```python
from build123d import *

# Parameters (mm, degrees)
F1_DEPTH = 40.2336
F2_DEPTH = 15.7734
F3_R     = 3.302


with BuildPart() as f1:
    # F0 (on Top) → F1 (new body)
    with BuildSketch(Plane.XY):
        with BuildLine():
            ThreePointArc((15.4849246273, -24.0155727453), (25.0899616005, -13.6756883515), (28.575, 0))
            ThreePointArc((28.575, 0), (24.3073468487, 15.0227665288), (12.7791284914, 25.5582569828))
            ThreePointArc((12.7791284914, 25.5582569828), (-28.532530963, -1.5573380643), (15.4849246273, -24.0155727453))
        make_face()
        with BuildLine():
            Line((18.5293, 4.826), (18.5293, 0))
            Line((18.5293, 0), (18.5293, -4.826))
            Line((18.5293, -4.826), (13.4477648793, -4.826))
            ThreePointArc((13.4477648793, -4.826), (-14.2875, 0), (13.4477648793, 4.826))
            Line((13.4477648793, 4.826), (18.5293, 4.826))
        make_face(mode=Mode.SUBTRACT)
    extrude(amount=F1_DEPTH)

    # F0 (on Top) → F2 (join)
    with BuildSketch(Plane.XY):
        with BuildLine():
            ThreePointArc((12.7791284914, 25.5582569828), (24.3073468487, 15.0227665288), (28.575, 0))
            Line((28.575, 0), (40.005, 0))
            ThreePointArc((40.005, 0), (44.0967182668, 9.8782817332), (53.975, 13.97))
            Line((53.975, 13.97), (12.7791284914, 25.5582569828))
        make_face()
        with BuildLine():
            Line((40.005, 0), (28.575, 0))
            ThreePointArc((28.575, 0), (25.0899616005, -13.6756883515), (15.4849246273, -24.0155727453))
            Line((15.4849246273, -24.0155727453), (53.975, -13.97))
            ThreePointArc((53.975, -13.97), (44.0967182668, -9.8782817332), (40.005, 0))
        make_face()
        with BuildLine():
            Line((46.355, 0), (40.005, 0))
            ThreePointArc((40.005, 0), (44.0967182668, -9.8782817332), (53.975, -13.97))
            Line((53.975, -13.97), (53.975, -7.62))
            ThreePointArc((53.975, -7.62), (48.5868463274, -5.3881536726), (46.355, 0))
        make_face()
        with BuildLine():
            ThreePointArc((53.975, 13.97), (44.0967182668, 9.8782817332), (40.005, 0))
            Line((40.005, 0), (46.355, 0))
            ThreePointArc((46.355, 0), (48.5868463274, 5.3881536726), (53.975, 7.62))
            Line((53.975, 7.62), (53.975, 13.97))
        make_face()
        with BuildLine():
            ThreePointArc((67.945, 0), (63.8532817332, 9.8782817332), (53.975, 13.97))
            Line((53.975, 13.97), (53.975, 7.62))
            ThreePointArc((53.975, 7.62), (59.3631536726, 5.3881536726), (61.595, 0))
            ThreePointArc((61.595, 0), (59.3631536726, -5.3881536726), (53.975, -7.62))
            Line((53.975, -7.62), (53.975, -13.97))
            ThreePointArc((53.975, -13.97), (63.8532817332, -9.8782817332), (67.945, 0))
        make_face()
    extrude(amount=F2_DEPTH)

    # F3
    f3_edges = [f1.edges().sort_by_distance(p)[0] for p in [
        (-15.484925, 24.015573, 40.2336),
    ]]
    fillet(f3_edges, radius=F3_R)


solid = f1.part
```
Source: CAD feature listing. Evaluate the final solid. Frame: model axes, mm. A direction names the side the tool comes from. Coordinates: 2 decimals unless noted, no trailing zeros. Loops run counter-clockwise (first coordinate to the right, second up) from the corner with the lowest first, then second, coordinate; pieces in that order, holes last. Notation, with made-up numbers: M -9,0.5 L -3,0.5 A22 ccw -3,19.5 Z; hole C 29.25,53.5 d2. An arc over 180 degrees is marked long. Put each result on its own line as item: value. Start each with the question number.
1) Contact query for flat-ended pins moving along their axis: pin 1 Ø4 at (x, z) = (15, 20.5) entering from +Y; pin 2 Ø25 at (x, y) = (31.5, -1) entering from +Z; pin 3 Ø4 at (x, z) = (15, 18.5) entering from -Y; pin 4 Ø4 at (y, z) = (-16, 34.5) entering from +X. Output: stop coordinate, or through.
2) Cut plane C-C on x = 40.5. Return the cut outline in (y, z).
3) Reachability of faces 4 (the face through (33.67, 19.68, 7.78)), 5 (the face through (16, -4.826, 20)) from +Z, -Z, +X, -X, +Y, -Y: full face, straight path, thin tool, end or side. Return the list, or none.
4) Pull-direction query (X, two-part tool) for faces 1 (the face through (19, 0, 0)), 2 (the face through (18.529, 0, 20)), 3 (the face through (34.461, -19.063, 7.776)); classes: pulls with the +X half, pulls with the -X half, needs draft (parallel to the pull), parting line crosses it, or undercut.
5) Cut plane B-B on z = 6. Give the number of separate pieces and of enclosed holes in the cut face, then the cut area to 3 significant figures.
6) Ray query, L1, parallel to X at y = -0.5, z = 9.5; L2, parallel to Y at x = 0, z = 30 (1 decimal); L3, parallel to X at y = 0, z = 18 (1 decimal). Return the intervals inside material, ascending. Write a range as from..to.
The answers:
1. pin 1: stops at y = 25.45
1. pin 2: stops at z = 40.23
1. pin 3: stops at y = -25.45
1. pin 4: stops at x = 24.91
2. outline: M -17.49,0 L 17.76,0 L 17.76,15.77 L -17.49,15.77 Z
3. face 4: +Z, -Z, +X, +Y
3. face 5: +Z, -Z
4. face 1: needs draft
4. face 2: undercut
4. face 3: pulls with the +X half
5. separate pieces: 1
5. enclosed holes: 2
5. area: 3,040 mm²
6. L1: x = -28.57..-14.28, 18.53..46.37, 61.58..67.94
6. L2: y = -28.6..-14.3, 14.3..28.6
6. L3: x = -28.6..-14.3, 18.5..28.6
